```python
from build123d import *

# Parameters (mm, degrees)
SKETCH1_R           = 1.6
SKETCH1_R_2         = 6
BOSS_EXTRUDE1_DEPTH = 5


with BuildPart() as part:
    # Sketch1 → Boss-Extrude1 (new body)
    with BuildSketch(Plane.XY):
        with BuildLine():
            Line((90, 30), (-90, 30))
            Line((-90, 30), (-104.760095102, 113.708659006))
            Line((-104.760095102, 113.708659006), (-122.253709396, 111.824739741))
            Line((-122.253709396, 111.824739741), (-129.926921508, 2.092694212))
            ThreePointArc((-129.926921508, 2.092694212), (-121.940611049, -20.459950802), (-100, -30))
            Line((-100, -30), (100, -30))
            ThreePointArc((100, -30), (121.940611049, -20.459950802), (129.926921508, 2.092694212))
            Line((129.926921508, 2.092694212), (122.253709396, 111.824739741))
            Line((122.253709396, 111.824739741), (104.760095102, 113.708659006))
            Line((104.760095102, 113.708659006), (90, 30))
        make_face()
        with Locations((-113.211659227, 101.998451941)):
            Circle(SKETCH1_R, mode=Mode.SUBTRACT)
        with Locations((-100, 0)):
            Circle(SKETCH1_R_2, mode=Mode.SUBTRACT)
        with Locations((100, 0)):
            Circle(SKETCH1_R_2, mode=Mode.SUBTRACT)
    extrude(amount=BOSS_EXTRUDE1_DEPTH)


solid = part.part
```
The model under review builds one solid part; all positions refer to its coordinate system, in mm. A direction names the side the tool comes from. Round coordinates to 2 decimals unless told otherwise and drop trailing zeros. Order: outer loops, then holes, each group sorted by start corner. A loop starts at its lowest first (then second) coordinate and runs counter-clockwise, first axis right, second up.
(1) Wall thickness on L1, parallel to X at y = 4, z = 3.7; L2, parallel to Y at x = -4.5, z = 4.65; L3, parallel to X at y = 74, z = 2.65: over which ranges is each line inside the solid? List them lowest first.
Working result:
L1: x = -129.79 to -104.47, -95.53 to 95.53, 104.47 to 129.79
L2: y = -30 to 30
L3: x = -124.9 to -97.76, 97.76 to 124.9
(2) For P1, Ø2, axis at y = -6, z = 3, coming from the -X side; P2, Ø1.5, axis at x = 44.5, z = 1.5, coming from the +Y side, all flat-tipped, find the tip position at first contact; note any pin that passes through.
Working result:
P1: stops at x = -129.58
P2: stops at y = 30
(3) Take a section at C-C, the plane x = 38.5. State the section outline as (y, z) points.
Working result:
outline: (-30, 0) - (30, 0) - (30, 5) - (-30, 5) - close
(4) Take a section at D-D, the plane y = 37.5. State the section outline as (x, z) points.
Working result:
outline: (-127.45, 0) - (-91.32, 0) - (-91.32, 5) - (-127.45, 5) - close; (91.32, 0) - (127.45, 0) - (127.45, 5) - (91.32, 5) - close
(5) Tool access review of faces 1 (the face through (113.629, 112.754, 2.465)), 2 (the face through (97.483, 72.44, 2.465)): name each direction out of +Z, -Z, +X, -X, +Y, -Y from which nothing blocks a thin tool from reaching the whole face with its end or side.
Working result:
face 1: +Z, -Z, +X, +Y
face 2: +Z, -Z, +Y
(6) Take a section at B-B, the plane z = 3.25. State the section outline as (x, y) points.
Working result:
outline: (-129.93, 2.09) arc R30 ccw to (-100, -30) - (100, -30) arc R30 ccw to (129.93, 2.09) - (122.25, 111.82) - (104.76, 113.71) - (90, 30) - (-90, 30) - (-104.76, 113.71) - (-122.25, 111.82) - close; hole circle Ø3.2 at (-113.21, 102); hole circle Ø12 at (-100, 0); hole circle Ø12 at (100, 0)
(7) Mouldability with a two-part tool opening along X and no side actions: class faces 3 (the face through (1, 30, 2)), 4 (the face through (-97.277, 71.268, 2.465)), 5 (the face through (-126.037, 57.727, 2.465)), 6 (the face through (121.704, -20.711, 2.465)) as released by +X, released by -X, zero draft, split by the parting line, or undercut.
Working result:
face 3: undercut
face 4: undercut
face 5: released by -X
face 6: released by +X
(8) Take a section at A-A, the plane y = 95.5. State the section outline as (x, z) points.
Working result:
outline: (-123.4, 0) - (-101.55, 0) - (-101.55, 5) - (-123.4, 5) - close; (101.55, 0) - (123.4, 0) - (123.4, 5) - (101.55, 5) - close
